Geometry: see drawing. Coordinates: mm, zero at the bounding-box minimum. A direction names the side the tool comes from. Round coordinates to 2 decimals unless told otherwise and drop trailing zeros. Write each loop counter-clockwise with the first axis right and the second up, starting at its lowest first coordinate (ties: lowest second). Pieces come first, ordered by that corner, then holes.
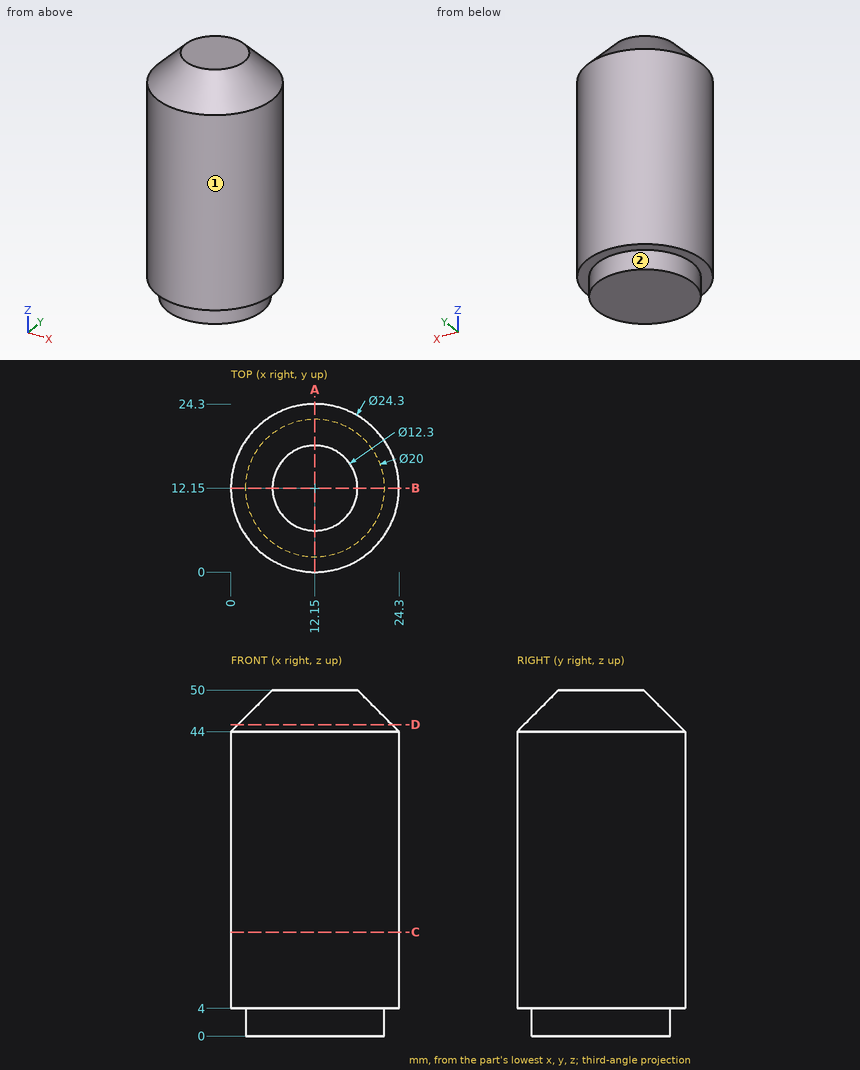
Q1. Section query A-A, the plane x = 12.15. Output: boundary loops of the cut face in (y, z), and give its area (3 significant figures).
Q2. Line query: line 1 (X direction, y = 11.75, z = 38); line 2 (Y direction, x = 12, z = 38); line 3 (X direction, y = 8.5, z = 38.5). Output: solid intervals per line, ascending.
Q3. Set-up query: the marked faces 1 and 2. Return all of +Z, -Z, +X, -X, +Y, -Y with unobstructed straight access to the full face (end or side cutting, diameter ignored); none if empty.
Q4. Section query D-D, the plane z = 45. Output: boundary loops of the cut face in (x, y), and give its area (3 significant figures).
Q5. Section query C-C, the plane z = 15. Output: boundary loops of the cut face in (x, y), and give its area (3 significant figures).
Q6. Pin query (flat end, axial travel): P1, Ø4, axis at y = 4, z = 7, coming from the -X side; P2, Ø1.5, axis at x = 17, z = 22.5, coming from the -Y side; P3, Ø12, axis at x = 17.5, y = 20, coming from the -Z side; P4, Ø3, axis at y = 17.5, z = 33.5, coming from the +X side. Return the tip coordinate at first contact, or that it passes through.
Filled in:
1. outline: (0, 4) - (2.15, 4) - (2.15, 0) - (22.15, 0) - (22.15, 4) - (24.3, 4) - (24.3, 44) - (18.3, 50) - (6, 50) - (0, 44) - close
1. area: 1,160 mm2
2. line 1: x = 0.01 to 24.29
2. line 2: y = 0 to 24.3
2. line 3: x = 0.56 to 23.74
3. face 1: +Z, -Z
3. face 2: -Z
4. outline: circle Ø22.3 at (12.15, 12.15)
4. area: 391 mm2
5. outline: circle Ø24.3 at (12.15, 12.15)
5. area: 464 mm2
6. P1: stops at x = 1.67
6. P2: stops at y = 0.71
6. P3: stops at z = 0
6. P4: stops at x = 23.67
